```python
from build123d import *

# Parameters (mm, degrees)
SKETCH1_W                   = 55.5
SKETCH1_H                   = 37.9
BRACKETBASE_DEPTH           = 2.5
SKETCH2_W                   = 7
SKETCH2_H                   = 20.5
SERVOMOUNTINGHOLETABS_DEPTH = 2.5
SKETCH3_R                   = 2.125
SERVOMOUNTINGHOLES_DEPTH    = 2.5
SKETCH4_W                   = 55.5
SKETCH4_H                   = 2.5
BASEWALL_DEPTH              = 23
SKETCH6_R                   = 5.7
BASETRIM_DEPTH              = 2.5
FILLET1_R                   = 2
SKETCH7_R                   = 2.125
M4MOUNTINGHOLE_DEPTH        = 10
SKETCH8_R                   = 2.125
CUT_EXTRUDE1_DEPTH          = 10
SKETCH9_R                   = 2.125
BOSS_EXTRUDE1_DEPTH         = 2.5
SKETCH10_R                  = 2.125
BOSS_EXTRUDE2_DEPTH         = 7.5


with BuildPart() as part:
    # Sketch1 → bracketBase (new body)
    with BuildSketch(Plane(origin=(0, 0, 0), x_dir=(1, 0, 0), z_dir=(0, 1, 0))):
        with Locations((27.75, 18.95)):
            Rectangle(SKETCH1_W, SKETCH1_H)
    extrude(amount=BRACKETBASE_DEPTH)

    # Sketch2 → servoMountingHoleTabs (add)
    with BuildSketch(Plane.XY.offset(-8.2)):
        with Locations((3.5, 12.75)):
            Rectangle(SKETCH2_W, SKETCH2_H)
        with Locations((52, 12.75)):
            Rectangle(SKETCH2_W, SKETCH2_H)
    extrude(amount=SERVOMOUNTINGHOLETABS_DEPTH)

    # Sketch3 → servoMountingHoles (cut)
    with BuildSketch(Plane.XY.offset(-5.7)):
        with Locations((3.75, 17.75)):
            Circle(SKETCH3_R)
        with Locations(Location((3.75, 7.75, 0), (0, 0, 180))):
            Circle(SKETCH3_R)
        with Locations((51.75, 7.75)):
            Circle(SKETCH3_R)
        with Locations(Location((51.75, 17.75, 0), (0, 0, 180))):
            Circle(SKETCH3_R)
    extrude(amount=-SERVOMOUNTINGHOLES_DEPTH, mode=Mode.SUBTRACT)

    # Sketch4 → baseWall (add)
    with BuildSketch(Plane(origin=(0, 0, 0), x_dir=(1, 0, 0), z_dir=(0, 1, 0))):
        with Locations((27.75, 39.15)):
            Rectangle(SKETCH4_W, SKETCH4_H)
    extrude(amount=BASEWALL_DEPTH)

    # Sketch6 → baseTrim (cut)
    with BuildSketch(Plane(origin=(0, 2.5, 0), x_dir=(1, 0, 0), z_dir=(0, 1, 0))):
        Circle(SKETCH6_R)
        with Locations((55.5, 0)):
            Circle(SKETCH6_R)
    extrude(amount=-BASETRIM_DEPTH, mode=Mode.SUBTRACT)

    # Fillet1
    fillet1_edges = [part.edges().sort_by_distance(p)[0] for p in [
        (0, 23, -6.95),
        (7, 23, -6.95),
        (55.5, 23, -6.95),
        (48.5, 23, -6.95),
        (55.5, 23, -39.15),
        (0, 23, -39.15),
    ]]
    fillet(fillet1_edges, radius=FILLET1_R)

    # Sketch7 → M4mountingHole (cut)
    with BuildSketch(Plane(origin=(0, 0, -40.4), x_dir=(-1, 0, 0), z_dir=(0, 0, -1))):
        with Locations((-17.25, 12.75)):
            Circle(SKETCH7_R)
    extrude(amount=-M4MOUNTINGHOLE_DEPTH, mode=Mode.SUBTRACT)

    # Sketch8 → Cut-Extrude1 (cut)
    with BuildSketch(Plane(origin=(0, 0, -40.4), x_dir=(-1, 0, 0), z_dir=(0, 0, -1))):
        with Locations((-38.25, 12.75)):
            Circle(SKETCH8_R)
    extrude(amount=-CUT_EXTRUDE1_DEPTH, mode=Mode.SUBTRACT)

    # Sketch9 → Boss-Extrude1 (add)
    with BuildSketch(Plane(origin=(0, 0, -40.4), x_dir=(-1, 0, 0), z_dir=(0, 0, -1))):
        with Locations((-17.25, 12.75)):
            Circle(SKETCH9_R)
    extrude(amount=-BOSS_EXTRUDE1_DEPTH)

    # Sketch10 → Boss-Extrude2 (add)
    # profile 1 of 2: a face of its own
    with BuildSketch(Plane(origin=(0, 0, -8.2), x_dir=(-1, 0, 0), z_dir=(0, 0, -1))):
        with BuildLine():
            Line((-48.5, 2.5), (-48.5, 21))
            ThreePointArc((-48.5, 21), (-49.085786438, 22.414213562), (-50.5, 23))
            Line((-50.5, 23), (-53.5, 23))
            ThreePointArc((-53.5, 23), (-54.914213562, 22.414213562), (-55.5, 21))
            Line((-55.5, 21), (-55.5, 2.5))
            Line((-55.5, 2.5), (-48.5, 2.5))
        make_face()
        with Locations((-51.75, 17.75)):
            Circle(SKETCH10_R, mode=Mode.SUBTRACT)
        with Locations(Location((-51.75, 7.75, 0), (0, 0, 180))):
            Circle(SKETCH10_R, mode=Mode.SUBTRACT)
    # profile 2 of 2: a face of its own
    with BuildSketch(Plane(origin=(0, 0, -8.2), x_dir=(-1, 0, 0), z_dir=(0, 0, -1))):
        with BuildLine():
            Line((-2, 23), (-5, 23))
            ThreePointArc((-5, 23), (-6.414213562, 22.414213562), (-7, 21))
            Line((-7, 21), (-7, 2.5))
            Line((-7, 2.5), (0, 2.5))
            Line((0, 2.5), (0, 21))
            ThreePointArc((0, 21), (-0.585786438, 22.414213562), (-2, 23))
        make_face()
        with Locations(Location((-3.75, 17.75, 0), (0, 0, 180))):
            Circle(SKETCH10_R, mode=Mode.SUBTRACT)
        with Locations((-3.75, 7.75)):
            Circle(SKETCH10_R, mode=Mode.SUBTRACT)
    extrude(amount=BOSS_EXTRUDE2_DEPTH)


solid = part.part
```
Check sheet for the modelled part. Datum: model origin and axes. Units: mm. A direction names the side the tool comes from. Give positions to 0.01 mm unless a question says otherwise; leave off trailing zeros. Write each loop counter-clockwise with the first axis right and the second up, starting at its lowest first coordinate (ties: lowest second). Pieces come first, ordered by that corner, then holes.
Item 1: Access from +Z, -Z, +X, -X, +Y, -Y to the whole of each face (thin tool, end or side, straight path). Record for faces 1 (the face through (52, 13, -15.7)), 2 (the face through (49.07, 22.4, -10.63)), 3 (the face through (52, 13, -5.7)).
Item 2: Cross-section at C-C (z = -7.5). Enter the section's corners in (x, y) (3 decimals).
Item 3: Cross-section at D-D (y = 4.5). Enter the section's corners in (x, z).
Item 4: Cross-section at A-A (x = 38.25). Enter the section's corners in (y, z) (3 decimals).
Item 5: Scan lines: L1, parallel to X at y = 17.75, z = -11.25 (3 decimals); L2, parallel to Y at x = 3.75, z = -6.35 (3 decimals); L3, parallel to Z at x = 49.5, y = 3.5. Record each from-to range of solid material in increasing order.
Item 6: Draft check along X on faces 4 (the face through (27, 1, 0)), 5 (the face through (48.5, 12, -11)), 6 (the face through (0.57, 22.4, -39.17)), 7 (the face through (27, 2.5, -19)). Enter one of: released by +X, released by -X, zero draft, split by the parting line, or undercut.
Item 7: Cross-section at B-B (y = 7.75). Enter the section's corners in (x, z) (3 decimals).
Item 8: Gauge pin test, flat ends, axial feed: pin 1 (5.5 mm diameter, centred on x = 3.75, y = 7.75, fed in from +Z); pin 2 (4 mm diameter, centred on x = 15, z = -32.5, fed in from +Y); pin 3 (4 mm diameter, centred on x = 46, y = 5.5, fed in from +Z). Record the tip position at first contact, or that the pin passes through.
Report:
1. face 1: +X, -X, +Y
1. face 2: +Z, +Y
1. face 3: +Z, +X, -X, +Y
2. outline: (0, 0) - (55.5, 0) - (55.5, 21) arc R2 ccw to (53.5, 23) - (50.5, 23) arc R2 ccw to (48.5, 21) - (48.5, 2.5) - (7, 2.5) - (7, 21) arc R2 ccw to (5, 23) - (2, 23) arc R2 ccw to (0, 21) - close; hole circle Ø4.25 at (3.75, 7.75); hole circle Ø4.25 at (3.75, 17.75); hole circle Ø4.25 at (51.75, 7.75); hole circle Ø4.25 at (51.75, 17.75)
3. outline: (0, -40.4) - (55.5, -40.4) - (55.5, -37.9) - (0, -37.9) - close; (0, -15.7) - (7, -15.7) - (7, -5.7) - (0, -5.7) - close; (48.5, -15.7) - (55.5, -15.7) - (55.5, -5.7) - (48.5, -5.7) - close
4. outline: (0, -40.4) - (10.625, -40.4) - (10.625, -37.9) - (2.5, -37.9) - (2.5, 0) - (0, 0) - close; (14.875, -40.4) - (23, -40.4) - (23, -37.9) - (14.875, -37.9) - close
5. L1: x = 0 to 1.625, 5.875 to 7, 48.5 to 49.625, 53.875 to 55.5
5. L2: y = 0 to 5.625, 9.875 to 15.625, 19.875 to 23
5. L3: z = -40.4 to -37.9, -15.7 to -5.7
6. face 4: zero draft
6. face 5: undercut
6. face 6: released by -X
6. face 7: undercut
7. outline: (0, -40.4) - (55.5, -40.4) - (55.5, -37.9) - (0, -37.9) - close; (0, -15.7) - (1.625, -15.7) - (1.625, -5.7) - (0, -5.7) - close; (5.875, -15.7) - (7, -15.7) - (7, -5.7) - (5.875, -5.7) - close; (48.5, -15.7) - (49.625, -15.7) - (49.625, -5.7) - (48.5, -5.7) - close; (53.875, -15.7) - (55.5, -15.7) - (55.5, -5.7) - (53.875, -5.7) - close
8. pin 1: stops at z = -5.7
8. pin 2: stops at y = 2.5
8. pin 3: stops at z = -37.9
